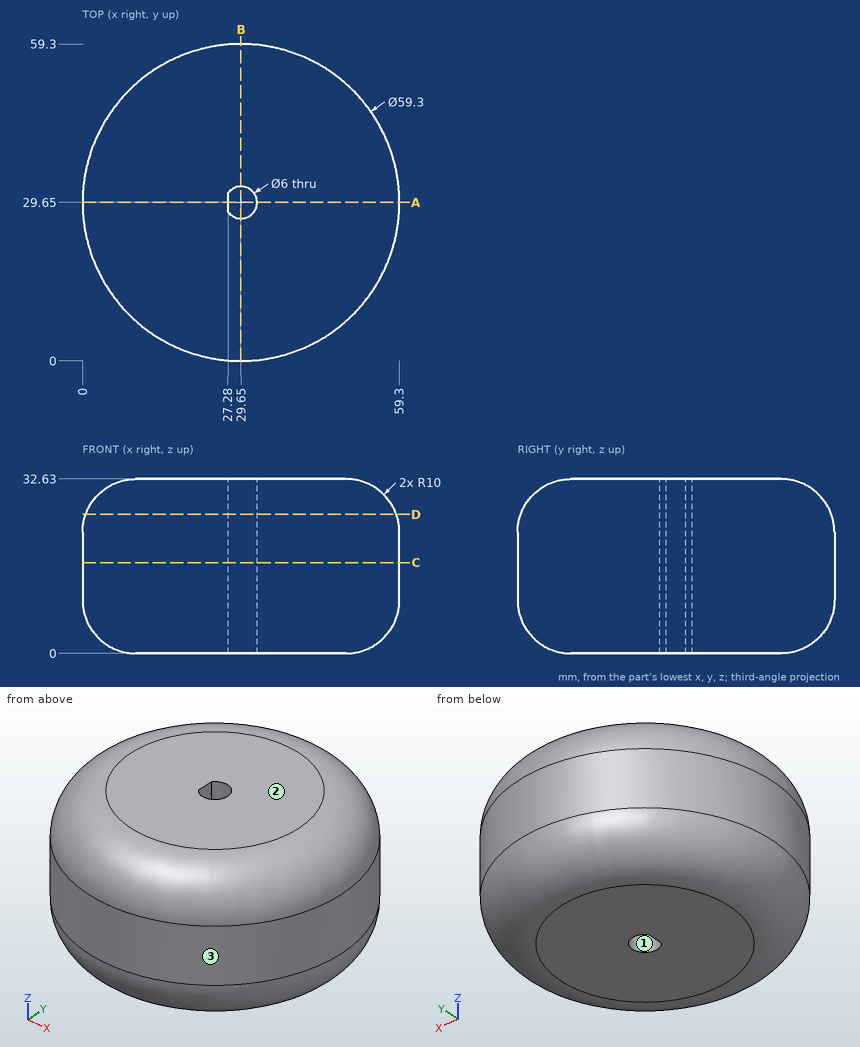
For this review, use the dimensioned drawing (mm, ordinates from the lowest corner) and the shaded views. Give positions to 0.01 mm unless a question says otherwise; leave off trailing zeros. Order: outer loops, then holes, each group sorted by start corner. A loop starts at its lowest first (then second) coordinate and runs counter-clockwise, first axis right, second up.
1) Wall thickness on line 1 (Y direction, x = 29.65, z = 15); line 2 (X direction, y = 29, z = 19); line 3 (Z direction, x = 7, y = 39): over which ranges is each line inside the solid? List them lowest first.
2) Take a section at D-D (z = 26). Give the boundary of the cut face in (x, y), then the cut area to 3 significant figures.
3) The part is to be moulded in two halves that separate along Y. For the marked faces 1, 2 and 3, say which applies: released by +Y, released by -Y, zero draft, split by the parting line, or undercut.
4) Take a section at B-B (x = 29.65). Give the boundary of the cut face in (y, z).
5) Insertion check: pin 1 (10 mm diameter, centred on y = 26.5, z = 4.5, fed in from +X); pin 2 (1 mm diameter, centred on x = 29.5, z = 27, fed in from -Y); pin 3 (4 mm diameter, centred on x = 11, y = 38.5, fed in from +Z); pin 4 (4 mm diameter, centred on y = 41.5, z = 11, fed in from -X). Each pin has a flat end and moves straight along its axis. Give the tip position at first contact, or say it passes through.
6) Take a section at A-A (y = 29.65). Give the boundary of the cut face in (x, z), then the cut area to 3 significant figures.
7) Take a section at C-C (z = 17). Give the boundary of the cut face in (x, y).
Derived:
1. line 1: y = 0 to 26.65, 32.65 to 59.3
1. line 2: x = 0.01 to 27.28, 32.58 to 59.29
1. line 3: z = 1.26 to 31.37
2. outline: circle Ø58.13 at (29.65, 29.65); hole (27.28, 27.81) arc R3 ccw (long way) to (27.28, 31.49) - close
2. area: 2,630 mm2
3. face 1: undercut
3. face 2: zero draft
3. face 3: split by the parting line
4. outline: (0, 10) arc R10 ccw to (10, 0) - (26.65, 0) - (26.65, 32.63) - (10, 32.63) arc R10 ccw to (0, 22.63) - close; (32.65, 0) - (49.3, 0) arc R10 ccw to (59.3, 10) - (59.3, 22.63) arc R10 ccw to (49.3, 32.63) - (32.65, 32.63) - close
5. pin 1: stops at x = 59.24
5. pin 2: stops at y = 0.78
5. pin 3: stops at z = 32.63
5. pin 4: stops at x = 1.68
6. outline: (0, 10) arc R10 ccw to (10, 0) - (27.28, 0) - (27.28, 32.63) - (10, 32.63) arc R10 ccw to (0, 22.63) - close; (32.65, 0) - (49.3, 0) arc R10 ccw to (59.3, 10) - (59.3, 22.63) arc R10 ccw to (49.3, 32.63) - (32.65, 32.63) - close
6. area: 1,670 mm2
7. outline: circle Ø59.3 at (29.65, 29.65); hole (27.28, 27.81) arc R3 ccw (long way) to (27.28, 31.49) - close
